```python
from build123d import *

# Parameters (mm, degrees)
F0_W      = 50.8
F0_H      = 50.8
F1_DEPTH  = 50.8
F4_DEPTH  = 58.6597873497
F5_R      = 6.35
F8_DEPTH  = 7.62
F6_R      = 3.175
F9_DEPTH  = 7.62
F7_R      = 1.5875
F10_DEPTH = 7.62


with BuildPart() as f1:
    # F0 (on Top) → F1 (new body)
    with BuildSketch(Plane.XY):
        Rectangle(F0_W, F0_H)
    extrude(amount=F1_DEPTH)

    # F3 (on 3pt) → F4 (cut, through all)
    with BuildSketch(Plane(origin=(16.9333333333, 16.9333333333, 16.9333333333), x_dir=(0.8164965809, -0.4082482905, -0.4082482905), z_dir=(-0.5773502692, -0.5773502692, -0.5773502692))):
        Polygon((-51.8475328889, 17.9605122421), (-31.1085197333, -17.9605122421), (10.3695065778, -17.9605122421), (31.1085197333, 17.9605122421), (10.3695065778, 53.8815367264), (-31.1085197333, 53.8815367264), align=None)
    extrude(amount=F4_DEPTH, mode=Mode.SUBTRACT)

    # F5 (on face) → F8 (cut)
    with BuildSketch(Plane.YZ.offset(25.4)):
        with Locations((8.4666666667, 33.8666666667)):
            Circle(F5_R)
    extrude(amount=-F8_DEPTH, mode=Mode.SUBTRACT)

    # F6 (on face) → F9 (cut)
    with BuildSketch(Plane.XY.offset(50.8)):
        with Locations((8.4666666667, 8.4666666667)):
            Circle(F6_R)
    extrude(amount=-F9_DEPTH, mode=Mode.SUBTRACT)

    # F7 (on face) → F10 (cut)
    with BuildSketch(Plane(origin=(0, 25.4, 0), x_dir=(-1, 0, 0), z_dir=(0, 1, 0))):
        with Locations((-8.4666666667, 33.8666666667)):
            Circle(F7_R)
    extrude(amount=-F10_DEPTH, mode=Mode.SUBTRACT)


solid = f1.part
```
Part model, mm, in its own coordinate system. A direction names the side the tool comes from. Give positions to 0.01 mm unless a question says otherwise; leave off trailing zeros. Order: outer loops, then holes, each group sorted by start corner. A loop starts at its lowest first (then second) coordinate and runs counter-clockwise, first axis right, second up. Notation, with made-up numbers: M 11,78.5 L 25,78.5 A21 ccw 25,102.5 Z; hole C 83.5,66 d3. An arc over 180 degrees is marked long. Use a Markdown table: item, result. Add a question column.
(1) Probe line 1 along Z through (x, y) = (22.5, 6.5); line 2 along X through (y, z) = (8.5, 27); line 3 along Z through (x, y) = (16, 22). List the from-to ranges inside material, lowest first. Write a range as [from, to].
(2) Saw through at B-B, the plane y = 3. Give the cut face in (x, z), and give its area (3 significant figures).
(3) Saw through at A-A, the plane z = 31. Give the cut face in (x, y), and give its area (3 significant figures).
(4) Drop flat-ended pins along their axis: P1, Ø3, axis at x = 9, y = 7.5, coming from the +Z side; P2, Ø3, axis at x = 14, z = 16.5, coming from the -Y side; P3, Ø4, axis at y = 7, z = 32.5, coming from the +X side. Give the stop position or say it passes through.
(5) Saw through at C-C, the plane x = -6. Give the cut face in (y, z), and give its area (3 significant figures).
(6) Mould opens along Y. For faces 4 (the face through (11, 12, 50.8)), 5 (the face through (5.3, 9.7, 35.8)), 6 (the face through (8, 9, 43.18)), 7 (the face through (11, 25.4, 36)) say: +Y half, -Y half, draft (parallel to the pull), parting line (faces both ways), or undercut.
(7) Saw through at D-D, the plane z = 46. Give the cut face in (x, y) (3 decimals).
(8) 3-axis set-ups, long thin cutter, end or side, ignore diameter. For faces 1 (the face through (9.637, 21.643, 34.94)), 2 (the face through (7.778, 5.367, 47.043)), 3 (the face through (21.643, 7.64, 40.163)): which of +Z, -Z, +X, -X, +Y, -Y reach the whole face in a straight line?
Answer key:
| question | item | result |
|---|---|---|
| 1 | line 1 | [21.8, 27.83], [39.9, 50.8] |
| 1 | line 2 | [15.3, 25.4] |
| 1 | line 3 | [12.8, 50.8] |
| 2 | outline | M -3,50.8 L 25.4,22.4 L 25.4,30.64 L 17.78,30.64 L 17.78,37.1 L 25.4,37.1 L 25.4,50.8 Z |
| 2 | area | 354 mm^2 |
| 3 | outline | M -5.6,25.4 L 25.4,-5.6 L 25.4,2.8 L 17.78,2.8 L 17.78,14.13 L 25.4,14.13 L 25.4,25.4 Z |
| 3 | area | 394 mm^2 |
| 4 | P1 | z = 43.18 |
| 4 | P2 | y = 18.18 |
| 4 | P3 | x = 17.78 |
| 5 | outline | M 6,50.8 L 25.4,31.4 L 25.4,50.8 Z |
| 5 | area | 188 mm^2 |
| 6 | face 4 | draft |
| 6 | face 5 | -Y half |
| 6 | face 6 | undercut |
| 6 | face 7 | +Y half |
| 7 | outline | M -20.6,25.4 L 25.4,-20.6 L 25.4,25.4 Z; hole C 8.467,8.467 d6.35 |
| 8 | face 1 | +Y |
| 8 | face 2 | +Z |
| 8 | face 3 | +X |
